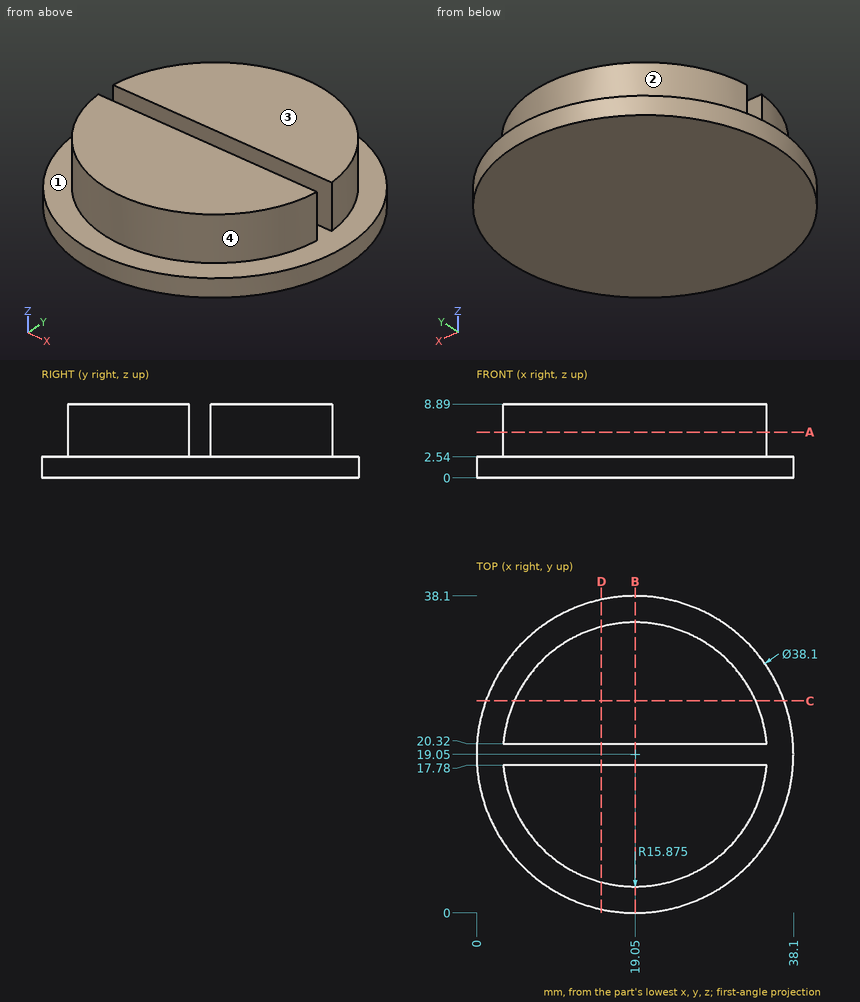
Verification items for this drawing (mm, ordinates from the low corner). Coordinates: 2 decimals unless noted, no trailing zeros. Loops run counter-clockwise (first coordinate to the right, second up) from the corner with the lowest first, then second, coordinate; pieces in that order, holes last. Notation, with made-up numbers: (9.25, 5) - (31.25, 5) arc R28 ccw to (31.25, 32) - close; hole circle Ø1 at (-39, 32). An arc over 180 degrees is marked (long way). One line per item, written item: value. Start each with the question number.
(1) Material ranges on line 1 (Y direction, x = 18.5, z = 4.5); line 2 (X direction, y = 18.5, z = 1); line 3 (Y direction, x = 5, z = 8.25), recorded low to high. Write a range as [from, to].
(2) Cross-section at A-A on z = 5.5. Enter the section's corners in (x, y) (3 decimals).
(3) Mould release check, pull along Y, two halves, no side actions. Record for the marked faces 1, 2, 3 and 4: released by +Y, released by -Y, zero draft, split by the parting line, or undercut.
(4) Cross-section at B-B on x = 19.05. Enter the section's corners in (y, z) (3 decimals), plus the area to 3 significant figures.
(5) Cross-section at C-C on y = 25.5. Enter the section's corners in (x, z).
(6) Depth check by flat-ended pin: P1, Ø1, axis at y = 15.5, z = 4, coming from the -X side; P2, Ø1.5, axis at x = 19, z = 2.5, coming from the +Y side; P3, Ø1.5, axis at y = 12.5, z = 4.5, coming from the -X side. Enter the tip coordinate at first touch or a pass-through.
(7) Cross-section at D-D on x = 15. Enter the section's corners in (y, z), plus the area to 3 significant figures.
Results below:
1. line 1: y = [3.18, 17.78], [20.32, 34.92]
1. line 2: x = [0.01, 38.09]
1. line 3: y = [11.66, 17.78], [20.32, 26.44]
2. outline: (3.226, 17.78) arc R15.875 ccw to (34.874, 17.78) - close; (3.226, 20.32) - (34.874, 20.32) arc R15.875 ccw to start
3. face 1: undercut
3. face 2: released by +Y
3. face 3: zero draft
3. face 4: released by -Y
4. outline: (0, 0) - (38.1, 0) - (38.1, 2.54) - (34.925, 2.54) - (34.925, 8.89) - (20.32, 8.89) - (20.32, 2.54) - (17.78, 2.54) - (17.78, 8.89) - (3.175, 8.89) - (3.175, 2.54) - (0, 2.54) - close
4. area: 282 mm2
5. outline: (1.13, 0) - (36.97, 0) - (36.97, 2.54) - (33.56, 2.54) - (33.56, 8.89) - (4.54, 8.89) - (4.54, 2.54) - (1.13, 2.54) - close
6. P1: stops at x = 3.47
6. P2: stops at y = 38.1
6. P3: stops at x = 4.27
7. outline: (0.44, 0) - (37.66, 0) - (37.66, 2.54) - (34.4, 2.54) - (34.4, 8.89) - (20.32, 8.89) - (20.32, 2.54) - (17.78, 2.54) - (17.78, 8.89) - (3.7, 8.89) - (3.7, 2.54) - (0.44, 2.54) - close
7. area: 273 mm2
